The model under review builds one solid part; all positions refer to its coordinate system, in mm. A direction names the side the tool comes from. Give positions to 0.01 mm unless a question says otherwise; leave off trailing zeros. Order: outer loops, then holes, each group sorted by start corner. A loop starts at its lowest first (then second) coordinate and runs counter-clockwise, first axis right, second up. Notation, with made-up numbers: (86, -16) - (91, -16) arc R18 cw to (91, -1) - close; hole circle Ø1 at (22, -15). An arc over 180 degrees is marked (long way). Use CSV: the item, a comma, the result in double quotes. Start each with the question number.
1. Take a section at A-A, the plane z = 11.5. Count the separate pieces of the cut face and the enclosed holes in it, then the cut area to 3 significant figures.
2. Take a section at D-D, the plane z = 3.25. State the section outline as (x, y) points.
3. Machinability: for faces 4 (the flat face through (62.865, 20, 13)), 5 (the flat face through (67, 24.13, 14)), 6 (the cylindrical face through (37.464, 32.206, 5.973)), which of the approach directions +Z, -Z, +X, -X, +Y, -Y give a long, thin tool a straight path to every point of the face, cutting with its end or side? Answer none if there is none.
4. Draft analysis for pull direction Y (two halves, no side actions). For faces 1 (the flat face through (73.406, 19, 9)), 2 (the cylindrical face through (9.2, 15.53, 13.91)), 3 (the cylindrical face through (58.555, 19.568, 5.973)), state which applies: released by +Y, released by -Y, zero draft, split by the parting line, or undercut.
5. To check wall thickness, follow line 1 (X direction, y = 19.05, z = 10.25) (3 decimals); line 2 (Z direction, x = 10.1, y = 19.05) (1 decimal); line 3 (Y direction, x = 24, z = 9.25). State the ranges of each line that lie inside material, in increasing order. Write a range as [from, to].
6. For pin 1 (8 mm diameter, centred on y = 26.5, z = 9, fed in from -X); pin 2 (1.8 mm diameter, centred on x = 8, y = 18.5, fed in from +Z) (3 decimals); pin 3 (7 mm diameter, centred on y = 19.5, z = 14, fed in from +X) (3 decimals); pin 4 (6 mm diameter, centred on y = 31.5, z = 13, fed in from -X), all flat-tipped, find the tip position at first contact; note any pin that passes through.
```python
from build123d import *

# Parameters (mm, degrees)
F0_W      = 73.406
F0_H      = 38.1
F1_DEPTH  = 9.525
F2_R      = 16.002
F3_R      = 3.96875
F3_W      = 7.62
F3_H      = 10.16
F4_DEPTH  = 8.89
F5_R      = 1.5875
F6_DEPTH  = 68.58
F7_R      = 1.778
F7_W      = 3.81
F7_H      = 6.35
F8_DEPTH  = 12.7
F9_R      = 7.62
F10_W     = 45.72
F10_H     = 28.575
F11_DEPTH = 5.08
F12_R     = 5.07999


# Not quite as in the source:
# - a fillet or chamfer is up to 0.001 mm smaller than in the source, because OpenCascade refuses the exact size


with BuildPart() as f1:
    # F0 (on Top) → F1 (new body)
    with BuildSketch(Plane.XY):
        with Locations((36.703, 19.05)):
            Rectangle(F0_W, F0_H)
    extrude(amount=F1_DEPTH)

    # F2
    f2_edges = [f1.edges().sort_by_distance(p)[0] for p in [
        (0, 38.1, 4.7625),
        (0, 0, 4.7625),
        (73.406, 38.1, 4.7625),
        (73.406, 0, 4.7625),
    ]]
    fillet(f2_edges, radius=F2_R)

    # F3 (on face) → F4 (join)
    with BuildSketch(Plane.XY.offset(9.525)):
        with Locations((7.366, 19.05)):
            Circle(F3_R)
        with Locations((66.675, 19.05)):
            Rectangle(F3_W, F3_H)
    extrude(amount=F4_DEPTH)

    # F5 (on face) → F6 (cut)
    with BuildSketch(Plane.YZ.offset(70.485)):
        with Locations((19.05, 14.605)):
            Circle(F5_R)
    extrude(amount=-F6_DEPTH, mode=Mode.SUBTRACT)

    # F7 (on face) → F8 (cut)
    with BuildSketch(Plane.XY.offset(18.415)):
        with Locations((7.366, 19.05)):
            Circle(F7_R)
        with Locations((66.675, 18.923)):
            Rectangle(F7_W, F7_H)
    extrude(amount=-F8_DEPTH, mode=Mode.SUBTRACT)

    # F9
    f9_edges = [f1.edges().sort_by_distance(p)[0] for p in [
        (36.703, 0, 0),
    ]]
    fillet(f9_edges, radius=F9_R)

    # F10 (on face) → F11 (cut)
    with BuildSketch(Plane.XY.offset(9.525)):
        with Locations((37.1440443242, 19.3675)):
            Rectangle(F10_W, F10_H)
    extrude(amount=-F11_DEPTH, mode=Mode.SUBTRACT)

    # F12 (radius 5.08 in the source; OpenCascade refuses exactly that, so slightly less here)
    f12_edges = [f1.edges().sort_by_distance(p)[0] for p in [
        (60.004044, 19.3675, 4.445),
        (37.144044, 33.655, 4.445),
        (14.284044, 19.3675, 4.445),
        (37.144044, 5.08, 4.445),
    ]]
    fillet(f12_edges, radius=F12_R)


solid = f1.part
```
Determined:
1,separate pieces,"2"
1,enclosed holes,"2"
1,area,"92.8 mm²"
2,outline,"(1.38, 16) arc R14.62 ccw to (16, 1.38) - (57.4, 1.38) arc R14.62 ccw to (72.03, 16) - (72.03, 22.1) arc R14.62 ccw to (57.4, 36.72) - (16, 36.72) arc R14.62 ccw to (1.38, 22.1) - close"
3,face 4,"+Z, +Y, -Y"
3,face 5,"+Z, +X, -X, +Y"
3,face 6,"+Z"
4,face 1,"zero draft"
4,face 2,"split by the parting line"
4,face 3,"undercut"
5,line 1,"x = [3.397, 5.588], [9.144, 11.335], [62.865, 64.77], [68.58, 70.485]"
5,line 2,"z = [0, 13], [16.2, 18.4]"
5,line 3,"y = [0, 5.09], [33.65, 38.1]"
6,pin 1,"stops at x = 0.01"
6,pin 2,"stops at z = 5.715"
6,pin 3,"stops at x = 70.485"
6,pin 4,"passes through"
